Autodesk Inventor part; units mm, degrees
ref_plane "YZ Plane" through (0, 0, 0) normal (1, 0, 0) x (0, 1, 0)
ref_plane "XZ Plane" through (0, 0, 0) normal (0, 1, 0) x (-1, 0, 0)
ref_plane "XY Plane" through (0, 0, 0) normal (0, 0, 1) x (1, 0, 0)
sketch "Sketch1" plane through (0, 0, 0) normal (0, 0, 1) x (1, 0, 0)
  circle A0 centre (8.602, 43.9333) radius 18.288 construction
  circle A1 centre (-28.4777, 18.849) radius 3.302
  circle A2 centre (0, 0) radius 3.302
  circle A3 centre (19.9674, 91.247) radius 3.302
  circle A4 centre (47.7138, 72.8821) radius 3.302
  ellipse E0 centre (12.1068, 49.2285) end of major axis (47.4715, 102.6587) minor radius 35.9584 construction
  circle A5 centre (8.602, 43.9333) radius 19.304
  circle A6 centre (8.602, 43.9333) radius 19.05 construction
  line L0 (47.4715, 102.6587) -> (-23.2579, -4.2018) construction
  line L1 (19.9674, 91.247) -> (47.4715, 102.6587) construction
  line L2 (47.7138, 72.8821) -> (47.4715, 102.6587) construction
  circle A7 centre (12.1068, 49.2285) radius 64.0738
  point P0 (0, 0)
  dimension "d3" = 38.1
  dimension "d4" = 0.254
extrude "Extrusion1" add sketch "Sketch1" along normal blind 2.286
equation "\"BendRadius\" = Thickness"
equation "\"BendReliefWidth\" = Thickness"
equation "\"BendReliefDepth\" = 0.5 * Thickness"
equation "\"CornerReliefSize\" = 4 * Thickness"
equation "\"MinimumRemnant\" = 2 * Thickness"
equation "\"TransitionRadius\" = BendRadius"
equation "\"JacobiRadiusSize\" = BendRadius"
equation "\"GapSize\" = Thickness"
properties part number "Upper Hub Plate" material "Aluminum"
For this review, take the finished solid that the model builds, in its own axes (mm). Coordinates: 2 decimals unless noted, no trailing zeros. Loops run counter-clockwise (first coordinate to the right, second up) from the corner with the lowest first, then second, coordinate; pieces in that order, holes last. Notation, with made-up numbers: (-34.75, 77) - (-23.75, 77) arc R25 cw to (-23.75, 105) - close; hole circle Ø6 at (69, -27.5). An arc over 180 degrees is marked (long way). Use a Markdown table: item, result. Add a question column.
Item 1: For line 1 (Y direction, x = 18, z = 2.05); line 2 (Y direction, x = 20, z = 1.6); line 3 (Y direction, x = -29.5, z = 0.1), list the stretches that pass through material, from the lowest coordinate up.
Item 2: We need section A-A (y = 0). Give the boundary of the cut face in (x, z), and give its area (3 significant figures).
Item 3: Mouldability with a two-part tool opening along X and no side actions: class faces 1 (the face through (41.673, 106.073, 1.127)), 2 (the face through (-31.777, 18.704, 1.127)), 3 (the face through (11, 64, 2.286)) as pulls with the +X half, pulls with the -X half, needs draft (parallel to the pull), parting line crosses it, or undercut.
Item 4: We need section D-D (y = 54.5). Give the boundary of the cut face in (x, z).
Item 5: We need section C-C (z = 1.9). Give the boundary of the cut face in (x, y), and give its area (3 significant figures).
Item 6: Insertion check: pin 1 Ø7.5 at (x, y) = (47.71, 72.88) entering from -Z; pin 2 Ø1 at (y, z) = (74.5, 1) entering from -X. Each pin has a flat end and moves straight along its axis. Give the tip position at first contact, or say it passes through.
Item 7: We need section B-B (x = 0). Give the boundary of the cut face in (y, z), and give its area (3 significant figures).
Results list:
| question | item | result |
|---|---|---|
| 1 | line 1 | y = -14.57 to 27.07, 60.8 to 88.6, 93.9 to 113.03 |
| 1 | line 2 | y = -14.36 to 28.35, 59.51 to 87.95, 94.55 to 112.81 |
| 1 | line 3 | y = 0.5 to 15.71, 21.99 to 97.96 |
| 2 | outline | (-28.91, 0) - (-3.3, 0) - (-3.3, 2.29) - (-28.91, 2.29) - close; (3.3, 0) - (53.12, 0) - (53.12, 2.29) - (3.3, 2.29) - close |
| 2 | area | 172 mm^2 |
| 3 | face 1 | parting line crosses it |
| 3 | face 2 | undercut |
| 3 | face 3 | needs draft |
| 4 | outline | (-51.75, 0) - (-7.55, 0) - (-7.55, 2.29) - (-51.75, 2.29) - close; (24.76, 0) - (75.96, 0) - (75.96, 2.29) - (24.76, 2.29) - close |
| 5 | outline | circle Ø128.15 at (12.11, 49.23); hole circle Ø6.6 at (-28.48, 18.85); hole circle Ø38.61 at (8.6, 43.93); hole circle Ø6.6 at (0, 0); hole circle Ø6.6 at (19.97, 91.25); hole circle Ø6.6 at (47.71, 72.88) |
| 5 | area | 11,600 mm^2 |
| 6 | pin 1 | stops at z = 0 |
| 6 | pin 2 | stops at x = -46.98 |
| 7 | outline | (-13.69, 0) - (-3.3, 0) - (-3.3, 2.29) - (-13.69, 2.29) - close; (3.3, 0) - (26.65, 0) - (26.65, 2.29) - (3.3, 2.29) - close; (61.21, 0) - (112.15, 0) - (112.15, 2.29) - (61.21, 2.29) - close |
| 7 | area | 194 mm^2 |
